Autodesk Inventor part; units mm, degrees
ref_plane "YZ Plane" through (0, 0, 0) normal (1, 0, 0) x (0, 1, 0)
ref_plane "XZ Plane" through (0, 0, 0) normal (0, 1, 0) x (-1, 0, 0)
ref_plane "XY Plane" through (0, 0, 0) normal (0, 0, 1) x (1, 0, 0)
sketch "スケッチ1" plane through (0, 0, 0) normal (0, 1, 0) x (-1, 0, 0)
  circle A0 centre (0, 0) radius 1.5
  line L0 (0, 0) -> (-21.2, 0) construction
  circle A1 centre (-21.2, 0) radius 1.5
  line L1 (0, 0) -> (-21.2, 0) construction
  line L2 (0, 3) -> (-21.2, 3)
  line L3 (-21.2, -3) -> (0, -3)
  arc A2 (0, -3) -> (0, 3) centre (0, 0) ccw
  arc A3 (-21.2, 3) -> (-21.2, -3) centre (-21.2, 0) ccw
  point P0 (-10.6, 0)
  dimension "d0" = 3
  dimension "d1" = 3
  dimension "d2" = 21.2
  dimension "d3" = 6
extrude "押し出し1" add sketch "スケッチ1" along normal blind 2
sketch "スケッチ2" plane through (0, 2, 0) normal (0, 1, 0) x (1, 0, 0)
  circle A0 centre (21.2, 0) radius 1.5
  circle A1 centre (0, 0) radius 1.5
  line L0 (0, -3) -> (21.2, -3)
  arc A2 (21.2, -3) -> (21.2, 3) centre (21.2, 0) ccw
  line L1 (21.2, 3) -> (0, 3)
  arc A3 (0, 3) -> (0, -3) centre (0, 0) ccw
  line L2 (3.3481, 1.02) -> (17.8519, 1.02)
  arc A4 (21.2, -1.5) -> (21.2, 1.5) centre (21.2, 0) ccw
  line L3 (17.8519, -1.02) -> (3.3481, -1.02)
  arc A5 (0, 1.5) -> (0, -1.5) centre (0, 0) ccw
  arc A6 (17.8519, 1.02) -> (17.8519, -1.02) centre (21.2, 0) ccw
  arc A7 (3.3481, -1.02) -> (3.3481, 1.02) centre (0, 0) ccw
  line L4 (0, -3) -> (21.2, -3)
  dimension "d8" = 1.98
  dimension "d12" = 1.98
  dimension "d13" = 2
  dimension "d14" = 2
extrude "押し出し2" cut sketch "スケッチ2" against normal blind 2 contours L2 A6 L3 A7
fillet "フィレット1" radius 1 4 edges at (3.3481, 1, 1.02) (3.3481, 1, -1.02) (17.8519, 1, 1.02) (17.8519, 1, -1.02)
properties part number "ウィングおさえ" material "ポリカーボネート、クリア"
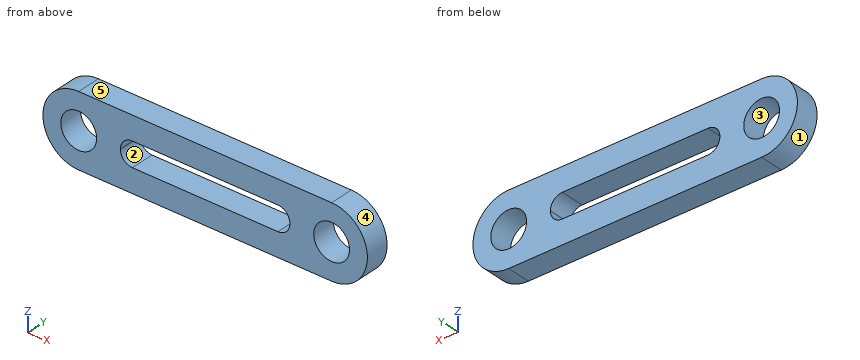
Work out the finished part from the listing and answer in its coordinate system (mm). Face numbers are marked on the shaded views. A direction names the side the tool comes from. Give positions to 0.01 mm unless a question says otherwise; leave off trailing zeros. Loops run counter-clockwise (first coordinate to the right, second up) from the corner with the lowest first, then second, coordinate; pieces in that order, holes last. Notation, with made-up numbers: (26.5, 40.5) -> (39.5, 40.5) arc R35 cw to (39.5, 72.5) -> close; hole circle Ø10 at (-32.75, -11.75). An arc over 180 degrees is marked (long way). Put each result on its own line as item: value. Start each with the question number.
Item 1: The part is cut by section C-C (x = 21.75). Give the vertices of the cut face in (y, z).
Item 2: The part is cut by section B-B (x = 17.25). Give the vertices of the cut face in (y, z), then the cut area to 3 significant figures.
Item 3: This flat-tipped pin is pushed along its axis until it touches: P1, Ø1.8, axis at x = 21.2, z = 0, coming from the +Y side. Where does it stop, or does it pass through?
Item 4: Find the intervals of material crossed by L1, parallel to X at y = 0.1, z = 0.25; L2, parallel to Z at x = 21.2, y = 1.35; L3, parallel to Z at x = 11.5, y = 0.8, in increasing order. Write a range as [from, to].
Item 5: The mould has two halves that part along X. Classify the marked faces 3, 4 and 5: released by +X, released by -X, zero draft, split by the parting line, or undercut.
Item 6: Which of the six approach directions +Z, -Z, +X, -X, +Y, -Y give full straight-line access (tool end or side, diameter ignored) to the marked faces 1 and 2?
Item 7: The part is cut by section A-A (y = 0.5). State how many separate pieces and enclosed holes the cut face has, then the cut area to 3 significant figures.
Answers below:
1. outline: (0, -2.95) -> (2, -2.95) -> (2, -1.4) -> (0, -1.4) -> close; (0, 1.4) -> (2, 1.4) -> (2, 2.95) -> (0, 2.95) -> close
2. outline: (0, -3) -> (2, -3) -> (2, -0.86) -> (0, -0.86) -> close; (0, 0.86) -> (2, 0.86) -> (2, 3) -> (0, 3) -> close
2. area: 8.58 mm2
3. P1: through
4. L1: [-2.99, -1.48], [1.48, 3.53], [17.67, 19.72], [22.68, 24.19]
4. L2: [-3, -1.5], [1.5, 3]
4. L3: [-3, -1.02], [1.02, 3]
5. face 3: undercut
5. face 4: released by +X
5. face 5: zero draft
6. face 1: -X, +Y, -Y
6. face 2: +Y, -Y
7. separate pieces: 1
7. enclosed holes: 3
7. area: 113 mm2
